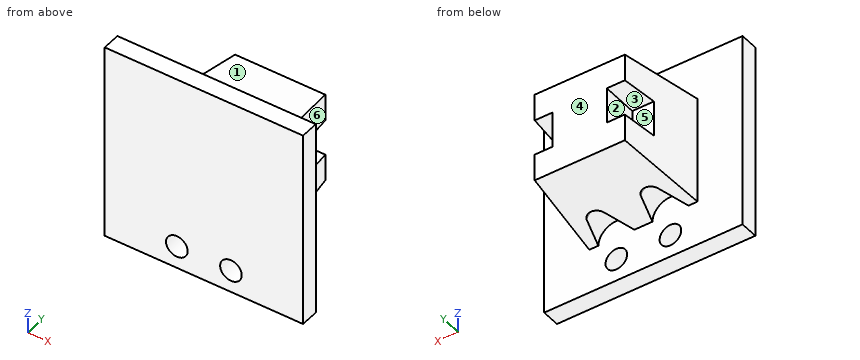
Solid Edge part; units mm, degrees
sketch "Sketch1" plane through (0, 0, 0) normal (0, -1, 0) x (1, 0, 0)
  line L0 (30, 30) -> (-30, 30)
  line L1 (-30, 30) -> (-30, -30)
  line L2 (-30, -30) -> (30, -30)
  line L3 (30, -30) -> (30, 30)
extrude "Protrusion1" add sketch "Sketch1" against normal blind 50
sketch "Sketch2" plane through (30, 25, 0) normal (1, 0, 0) x (0, 0, -1)
  line L0 (30, 25) -> (25, 25)
  line L1 (25, 25) -> (30, -25)
  line L2 (30, -25) -> (30, 25)
extrude "ExtrudedCutout_1" cut sketch "Sketch2" against normal blind 60 and the other way blind 1
sketch "Sketch3" plane through (30, 25, 0) normal (1, 0, 0) x (0, 0, -1)
  line L0 (-30, 25) -> (-30, -25)
  line L1 (-25, 25) -> (-30, -25)
  line L2 (-30, 25) -> (-25, 25)
extrude "ExtrudedCutout_2" cut sketch "Sketch3" against normal blind 60 and the other way blind 1
extrude "Protrusion2" [suppressed]
sketch "Sketch4" plane through (0, 25, -35) normal (0, 0, -1) x (-1, 0, 0)
  line L0 (30, 25) -> (25, 25)
  line L1 (25, 25) -> (30, -25)
  line L2 (30, -25) -> (30, 25)
extrude "ExtrudedCutout_3" cut sketch "Sketch4" against normal blind 65 and the other way blind 1
sketch "Sketch5" plane through (0, 25, -35) normal (0, 0, -1) x (-1, 0, 0)
  line L0 (-30, -25) -> (-30, 25)
  line L1 (-30, 25) -> (-25, 25)
  line L2 (-25, 25) -> (-30, -25)
extrude "ExtrudedCutout_4" cut sketch "Sketch5" against normal blind 65 and the other way blind 1
sketch "Sketch6" plane through (0, 50, 0) normal (0, 1, 0) x (1, 0, 0)
  line L0 (15, -10) -> (25, -10)
  line L1 (15, 10) -> (15, -10)
  line L2 (25, 10) -> (15, 10)
  line L3 (25, 10) -> (30, 10)
  line L4 (30, 10) -> (30, -10)
  line L5 (30, -10) -> (25, -10)
extrude "ExtrudedCutout_5" cut sketch "Sketch6" against normal blind 20 and the other way blind 1
sketch "Sketch7" plane through (0, 50, 0) normal (0, 1, 0) x (0, 0, -1)
  line L0 (10, 25) -> (10, 15)
  line L1 (10, 15) -> (-10, 15)
  line L2 (-10, 15) -> (-10, 30)
  line L3 (-10, 30) -> (10, 30)
  line L4 (10, 30) -> (10, 25)
extrude "ExtrudedCutout_6" cut sketch "Sketch7" against normal blind 20 and the other way blind 1
sketch "Sketch8" plane through (0, 25, -27.5) normal (0, 0.0995, -0.995) x (-1, 0, 0)
  line L0 (-15, -25.1247) -> (-15, -10.1247)
  line L1 (-15, -10.1247) -> (-15, -5.1247)
  line L2 (-25, -25.1247) -> (-19.7663, -8.6138)
  line L3 (-25, -25.1247) -> (-15, -25.1247)
  arc A0 (-19.7663, -8.6139) -> (-15, -5.1246) centre (-15, -10.1246) cw
revolve "RevolvedCutout_1" cut sketch "Sketch8" angle 180 about axis through (15, 0, -30) along (0, -0.995, -0.0995)
sketch "Sketch9" plane through (0, 25, -27.5) normal (0, 0.0995, -0.995) x (-1, 0, 0)
  line L0 (25, -25.1247) -> (19.7728, -8.6345)
  line L1 (25, -25.1247) -> (15, -25.1247)
  line L2 (15, -25.1247) -> (15, -10.1247)
  line L3 (15, -10.1247) -> (15, -5.1247)
  arc A0 (15, -5.1246) -> (19.7728, -8.6346) centre (15, -10.1246) cw
revolve "RevolvedCutout_2" cut sketch "Sketch9" angle 180 about axis through (-15, 0, -30) along (0, 0.995, 0.0995)
sketch "Sketch10" plane through (0, 0, 0) normal (0, -1, 0) x (0, 0, 1)
  line L0 (55, 55) -> (-55, 55)
  line L1 (-55, 55) -> (-55, -55)
  line L2 (-55, -55) -> (55, -55)
  line L3 (55, -55) -> (55, 55)
extrude "ExtrudedProtrusion_4" add sketch "Sketch10" along normal blind 10
sketch "Sketch11" plane through (0, 0, 0) normal (0, 1, 0) x (1, 0, 0)
  circle A0 centre (15, 42.5) radius 6
  circle A1 centre (-15, 42.5) radius 6
extrude "ExtrudedCutout_8" cut sketch "Sketch11" against normal blind 10 and the other way blind 1
Geometry check sheet. Reference: the model listing, model coordinates, mm. Face numbers are marked on the shaded views. A direction names the side the tool comes from. Coordinates: 2 decimals unless noted, no trailing zeros. Write each loop counter-clockwise with the first axis right and the second up, starting at its lowest first coordinate (ties: lowest second). Pieces come first, ordered by that corner, then holes. Notation, with made-up numbers: M 34.5,34 L 45.5,34 A26 ccw 45.5,72 Z; hole C -3.5,88.5 d6. An arc over 180 degrees is marked long. Use one line per item in the form item = value. Start each with the question number.
1) Release check for a two-part mould opening along Z. For the marked faces 1, 2, 3 and 4 record: pulls with the +Z half, pulls with the -Z half, needs draft (parallel to the pull), parting line crosses it, or undercut.
2) Section check B-B on z = -14. Enter the section's corners in (x, y), and give its area (3 significant figures).
3) Set-up check for the marked faces 5 and 6: record each of +Z, -Z, +X, -X, +Y, -Y from which the full face is reachable in a straight line by a thin tool's end or side.
4) Thickness scan on probe 1 along X at (y, z) = (-7, -42); probe 2 along Z at (x, y) = (15, -3.5); probe 3 along Y at (x, z) = (38, -13). Record the ranges inside material, lowest first. Write a range as from..to.
5) Go/stop test with flat-tipped pins: pin 1 Ø1.5 at (y, z) = (29, 4) entering from +X (3 decimals); pin 2 Ø22 at (y, z) = (40.5, 0) entering from +X; pin 3 Ø10 at (x, z) = (40.5, -32.5) entering from +Y. Record where each tip stops, or that it passes through.
6) Section check C-C on y = 18. Enter the section's corners in (x, z), and give its area (3 significant figures).
7) Section check A-A on z = -42.5. Enter the section's corners in (x, y).
8) Section check D-D on x = 40. Enter the section's corners in (y, z).
Responses:
q1.face_1 = pulls with the +Z half
q1.face_2 = undercut
q1.face_3 = undercut
q1.face_4 = needs draft
q2.outline = M -55,-10 L 55,-10 L 55,0 L 30,0 L 25,50 L -25,50 L -30,0 L -55,0 Z
q2.area = 3,850 mm2
q3.face_5 = -X, +Y
q3.face_6 = +Z, -Z, +X, +Y
q4.probe_1 = -55..-20.98, -9.02..9.02, 20.98..55
q4.probe_2 = -55..-48.5, -36.5..55
q4.probe_3 = -10..0
q5.pin_1 = 27.175
q5.pin_2 = 27.05
q5.pin_3 = 0
q6.outline = M -28.2,-28.2 L -18.93,-28.2 A3.94 cw -11.07,-28.2 L 11.07,-28.2 A3.94 cw 18.93,-28.2 L 28.2,-28.2 L 28.2,28.2 L -28.2,28.2 Z
q6.area = 3,140 mm2
q7.outline = M -55,-10 L -21,-10 L -21,0 L -55,0 Z; M -9,-10 L 9,-10 L 9,0 L -9,0 Z; M 21,-10 L 55,-10 L 55,0 L 21,0 Z
q8.outline = M -10,-55 L 0,-55 L 0,55 L -10,55 Z
